Geometry: see drawing. Coordinates: mm, zero at the bounding-box minimum. A direction names the side the tool comes from. Give positions to 0.01 mm unless a question says otherwise; leave off trailing zeros. Write each loop counter-clockwise with the first axis right and the second up, starting at its lowest first coordinate (ties: lowest second). Pieces come first, ordered by that corner, then holes. Notation, with made-up numbers: (45, 56) - (88, 56) arc R19 cw to (88, 74) - close; hole circle Ø10 at (30, 40). An arc over 180 degrees is marked (long way). Use a Markdown table: item, result. Add a question column.
1. Section query D-D, the plane y = 26. Return loops of the section in (x, z).
2. Material intervals for probe 1 along Z at (x, y) = (9, 11); probe 2 along Y at (x, z) = (6, 13); probe 3 along X at (y, z) = (22, 21.5), sorted ascending.
3. Section query A-A, the plane y = 17.5. Return loops of the section in (x, z).
4. Section query B-B, the plane x = 42. Return loops of the section in (y, z).
5. Pin query (flat end, axial travel): pin 1 (9.5 mm diameter, centred on y = 11, z = 25.5, fed in from -X); pin 2 (10 mm diameter, centred on x = 11, y = 20.5, fed in from -Z); pin 3 (5.5 mm diameter, centred on x = 12.5, y = 10, fed in from +Z); pin 4 (9.5 mm diameter, centred on y = 12.5, z = 24, fed in from +X). Return the tip coordinate at first contact, or that it passes through.
6. Section query C-C, the plane z = 25.5. Return loops of the section in (x, y).
7. Set-up query: the marked faces 1, 2 and 3. Return all of +Z, -Z, +X, -X, +Y, -Y with unobstructed straight access to the full face (end or side cutting, diameter ignored); none if empty.
8. Mould query, pull axis X, two halves, no side actions, for the marked faces 4, 5 and 6. Classes: released by +X, released by -X, zero draft, split by the parting line, or undercut.
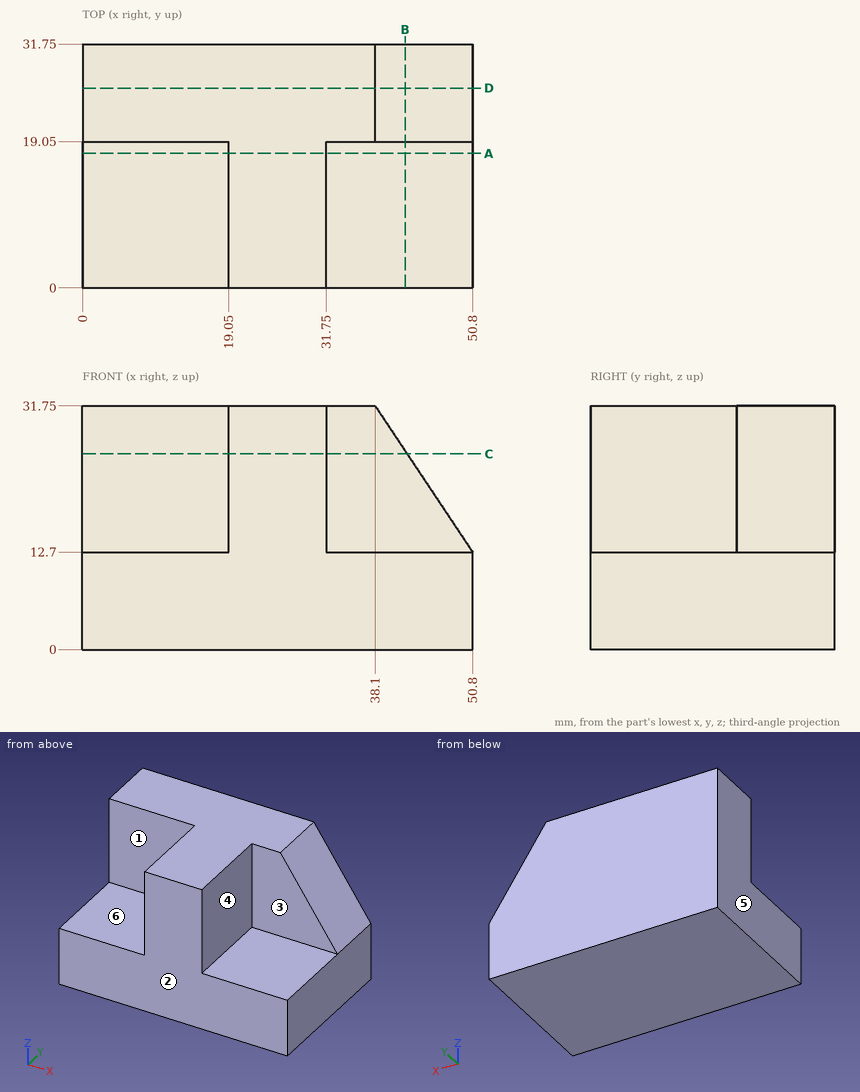
Result sheet:
| question | item | result |
|---|---|---|
| 1 | outline | (0, 0) - (50.8, 0) - (50.8, 12.7) - (38.1, 31.75) - (0, 31.75) - close |
| 2 | probe 1 | z = 0 to 12.7 |
| 2 | probe 2 | y = 19.05 to 31.75 |
| 2 | probe 3 | x = 0 to 44.93 |
| 3 | outline | (0, 0) - (50.8, 0) - (50.8, 12.7) - (31.75, 12.7) - (31.75, 31.75) - (19.05, 31.75) - (19.05, 12.7) - (0, 12.7) - close |
| 4 | outline | (0, 0) - (31.75, 0) - (31.75, 25.9) - (19.05, 25.9) - (19.05, 12.7) - (0, 12.7) - close |
| 5 | pin 1 | stops at x = 19.05 |
| 5 | pin 2 | stops at z = 0 |
| 5 | pin 3 | stops at z = 12.7 |
| 5 | pin 4 | stops at x = 31.75 |
| 6 | outline | (0, 19.05) - (19.05, 19.05) - (19.05, 0) - (31.75, 0) - (31.75, 19.05) - (42.27, 19.05) - (42.27, 31.75) - (0, 31.75) - close |
| 7 | face 1 | +Z, -X, -Y |
| 7 | face 2 | +Z, -Z, +X, -X, -Y |
| 7 | face 3 | +Z, +X, -Y |
| 8 | face 4 | released by +X |
| 8 | face 5 | released by -X |
| 8 | face 6 | zero draft |
